```python
from build123d import *

# Parameters (mm, degrees)
F0_W     = 205.173201859
F0_H     = 156.0566946864
F1_DEPTH = 94.996
F2_W     = 175.066800788
F2_H     = 135.7703600079
F3_DEPTH = 115.57
F4_R     = 27.2832059301
F5_DEPTH = 205.174201859
F6_W     = 113.4773865342
F6_H     = 60.8573002977
F7_DEPTH = 156.0576946864


with BuildPart() as f1:
    # F0 (on Top) → F1 (new body)
    with BuildSketch(Plane.XY):
        with Locations((10.3972144425, -9.1738365591)):
            Rectangle(F0_W, F0_H)
    extrude(amount=F1_DEPTH)

    # F2 (on face) → F3 (cut)
    with BuildSketch(Plane.XY.offset(94.996)):
        with Locations((11.4888912067, -10.3168571368)):
            Rectangle(F2_W, F2_H)
    extrude(amount=-F3_DEPTH, mode=Mode.SUBTRACT)

    # F4 (on face) → F5 (cut, through all)
    with BuildSketch(Plane.YZ.offset(112.983815372)):
        with Locations((-9.1738365591, 47.498)):
            Circle(F4_R)
    extrude(amount=-F5_DEPTH, mode=Mode.SUBTRACT)

    # F6 (on face) → F7 (cut, through all)
    with BuildSketch(Plane.XZ.offset(87.2021839023)):
        with Locations((10.3972144425, 94.996)):
            Rectangle(F6_W, F6_H)
    extrude(amount=-F7_DEPTH, mode=Mode.SUBTRACT)


solid = f1.part
```
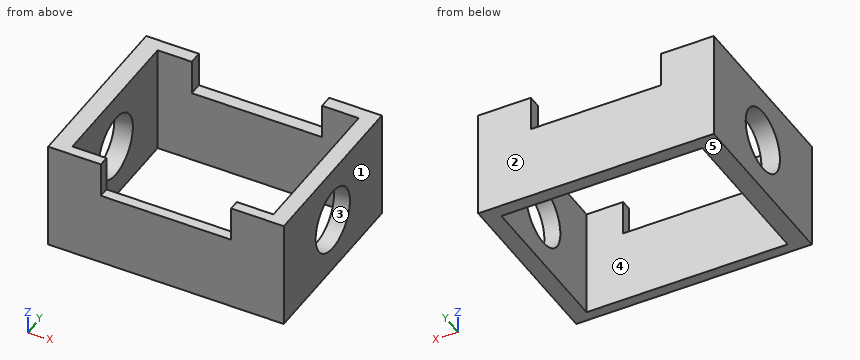
The listing builds one solid part. Answer for the finished solid, in the listing's coordinates (mm). Face numbers are marked on the shaded views. A direction names the side the tool comes from. Give positions to 0.01 mm unless a question says otherwise; leave off trailing zeros. Loops run counter-clockwise (first coordinate to the right, second up) from the corner with the lowest first, then second, coordinate; pieces in that order, holes last. Notation, with made-up numbers: (-3, -10.5) - (37, -10.5) arc R23 ccw to (37, 0.5) - close; hole circle Ø9 at (13.5, -6). An arc over 180 degrees is marked (long way). Return JSON: item names as keys, results as strings. Group by question number.
1. Find section B-B (x = 43.5). Write down the section's boundary in (y, z), then the cut area to 3 significant figures.
2. Determine the mould class of the marked faces 1, 2 and 3 for opening direction Y: pulls with the +Y half, pulls with the -Y half, needs draft (parallel to the pull), parting line crosses it, or undercut.
3. Find section A-A (z = 85.5). Write down the section's boundary in (x, y).
4. Find section D-D (z = 8.5). Write down the section's boundary in (x, y).
5. Straight lines are drawn through the part: line 1 (X direction, y = -15, z = 12.5); line 2 (Y direction, x = 84, z = 8); line 3 (X direction, y = -79.5, z = 90.5). For each, find the intervals that lie inside material, in ascending order. Write a range as [from, to].
6. Find section C-C (y = -45). Write down the section's boundary in (x, z), then the cut area to 3 significant figures.
7. Given pin 1 Ø6 at (x, z) = (-22, 67) entering from +Y; pin 2 Ø3.5 at (x, y) = (-10.5, 61) entering from +Z, each flat-ended and moving along its own axis, determine where each tip first touches the part or whether it passes through.
8. Which of the six approach directions +Z, -Z, +X, -X, +Y, -Y give full straight-line access (tool end or side, diameter ignored) to the marked faces 4 and 5?
Verdict:
{
 "1": {"outline": "(-87.2, 0) - (-78.2, 0) - (-78.2, 64.57) - (-87.2, 64.57) - close; (57.57, 0) - (68.85, 0) - (68.85, 64.57) - (57.57, 64.57) - close", "area": "1,310 mm^2"},
 "2": {"face 1": "needs draft", "face 2": "pulls with the +Y half", "face 3": "undercut"},
 "3": {"outline": "(-92.19, -87.2) - (-46.34, -87.2) - (-46.34, -78.2) - (-76.04, -78.2) - (-76.04, 57.57) - (-46.34, 57.57) - (-46.34, 68.85) - (-92.19, 68.85) - close; (67.14, -87.2) - (112.98, -87.2) - (112.98, 68.85) - (67.14, 68.85) - (67.14, 57.57) - (99.02, 57.57) - (99.02, -78.2) - (67.14, -78.2) - close"},
 "4": {"outline": "(-92.19, -87.2) - (112.98, -87.2) - (112.98, 68.85) - (-92.19, 68.85) - close; hole (-76.04, -78.2) - (99.02, -78.2) - (99.02, 57.57) - (-76.04, 57.57) - close"},
 "5": {"line 1": "x = [-92.19, -76.04], [99.02, 112.98]", "line 2": "y = [-87.2, -78.2], [57.57, 68.85]", "line 3": "x = [-92.19, -46.34], [67.14, 112.98]"},
 "6": {"outline": "(-92.19, 0) - (-76.04, 0) - (-76.04, 95) - (-92.19, 95) - close; (99.02, 0) - (112.98, 0) - (112.98, 95) - (99.02, 95) - close", "area": "2,860 mm^2"},
 "7": {"pin 1": "stops at y = 68.85", "pin 2": "stops at z = 64.57"},
 "8": {"face 4": "+Z, -Z", "face 5": "-Z, +X, -X, +Y, -Y"}
}
